Could you check a few things on this model? Use its own coordinates, in mm. Face numbers are marked on the shaded views. A direction names the side the tool comes from. Give positions to 0.01 mm unless a question says otherwise; leave off trailing zeros. Loops run counter-clockwise (first coordinate to the right, second up) from the corner with the lowest first, then second, coordinate; pieces in that order, holes last. Notation, with made-up numbers: M 28,-1 L 38,-1 A22 ccw 38,25 Z; hole C 22.25,34 d7. An arc over 180 degrees is marked long. Use a Markdown table: item, result. Add a question column.
1) Suppose I cut it at C-C on z = 17.5. List the corners of the cut face in (x, y) for me, and give its area (3 significant figures).
2) We'd pull the mould along Z, two halves only. Please class the marked faces 1, 2 and 3: +Z half, -Z half, draft (parallel to the pull), parting line (faces both ways), or undercut.
3) Which directions (+Z, -Z, +X, -X, +Y, -Y) give clear straight access to the entire face, cutting with the end or side of a thin tool? Please do the marked faces 4 and 5.
4) Suppose I cut it at B-B on x = 16.25. List the corners of the cut face in (y, z) for me, and give its area (3 significant figures).
5) Suppose I cut it at D-D on y = 5.5. List the corners of the cut face in (x, z) for me, and give its area (3 significant figures).
6) If I drill on line 1 along Z through (x, y) = (17.75, 4.75); line 2 along Y through (x, z) = (4.5, 28); line 3 along X through (y, z) = (6.25, 4.5), over which ranges is the centre line in solid material (lowest first)? Write a range as [from, to].
7) Suppose I cut it at A-A on z = 5. List the corners of the cut face in (x, y) for me.
8) Will these pins go through, and if not, where does the flat tip stop? pin 1 Ø2 at (y, z) = (6, 15.5) entering from +X; pin 2 Ø1 at (y, z) = (6, 6.5) entering from +X; pin 3 Ø5.5 at (x, z) = (1.5, 11) entering from +Y.
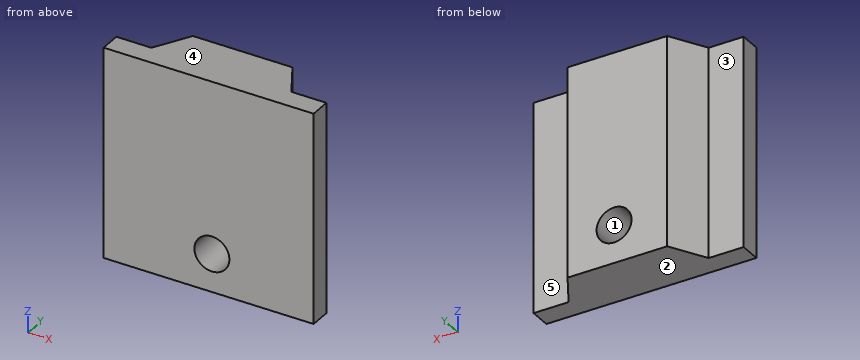
```python
from build123d import *

# Parameters (mm, degrees)
SKETCH_1_W          = 30
SKETCH_1_H          = 8
EXTRUDE_1_DEPTH     = 30
CUT_EXTRUDE_2_DEPTH = 44.17406629
M6X1_01_D           = 5
M6X1_01_DEPTH       = 17
M6X1_01_TIP         = 1.502151548


with BuildPart() as part:
    # Эскиз1 → Бобышка-Вытянуть1 (new body)
    with BuildSketch(Plane.XY):
        with Locations((15, 4)):
            Rectangle(SKETCH_1_W, SKETCH_1_H)
    extrude(amount=EXTRUDE_1_DEPTH)

    # Эскиз3 → Вырез-Вытянуть2 (cut, through all)
    with BuildSketch(Plane.XY.offset(30)):
        Polygon((5, 3), (7.886751346, 8), (5, 8), (0, 8), (0, 3), align=None)
        Polygon((25, 3), (30, 3), (30, 8), (25, 8), (22.113248654, 8), align=None)
    extrude(amount=-CUT_EXTRUDE_2_DEPTH, mode=Mode.SUBTRACT)

    # Отверстие обработанное метчиком M6x1.01
    with Locations(Plane(origin=(0, 8, 0), x_dir=(1, 0, 0), z_dir=(0, 1, 0))):
        with Locations((15.468545431, -5.425177516)):
            Hole(M6X1_01_D / 2, depth=M6X1_01_DEPTH)
            with Locations((0, 0, -(M6X1_01_DEPTH + M6X1_01_TIP / 2))):  # 118° drill point
                Cone(0, M6X1_01_D / 2, M6X1_01_TIP, mode=Mode.SUBTRACT)


solid = part.part
```
Answer block:
| question | item | result |
|---|---|---|
| 1 | outline | M 0,0 L 30,0 L 30,3 L 25,3 L 22.11,8 L 7.89,8 L 5,3 L 0,3 Z |
| 1 | area | 176 mm^2 |
| 2 | face 1 | undercut |
| 2 | face 2 | -Z half |
| 2 | face 3 | draft |
| 3 | face 4 | +Z, +X, -X, +Y, -Y |
| 3 | face 5 | +Z, -Z, +X, +Y |
| 4 | outline | M 0,0 L 8,0 L 8,3.05 L 0,3.05 Z; M 0,7.8 L 8,7.8 L 8,30 L 0,30 Z |
| 4 | area | 202 mm^2 |
| 5 | outline | M 6.44,0 L 23.56,0 L 23.56,30 L 6.44,30 Z; hole C 15.47,5.43 d5 |
| 5 | area | 494 mm^2 |
| 6 | line 1 | z = [0, 4.4], [6.45, 30] |
| 6 | line 2 | y = [0, 3] |
| 6 | line 3 | x = [6.88, 13.15], [17.79, 23.12] |
| 7 | outline | M 0,0 L 13,0 L 13,8 L 7.89,8 L 5,3 L 0,3 Z; M 17.93,0 L 30,0 L 30,3 L 25,3 L 22.11,8 L 17.93,8 Z |
| 8 | pin 1 | stops at x = 23.85 |
| 8 | pin 2 | stops at x = 23.56 |
| 8 | pin 3 | stops at y = 3 |
